Here's how the part is built. I have some questions about the finished solid (model axes, mm). A direction names the side the tool comes from. Coordinates: 2 decimals unless noted, no trailing zeros. Order: outer loops, then holes, each group sorted by start corner. A loop starts at its lowest first (then second) coordinate and runs counter-clockwise, first axis right, second up. Notation, with made-up numbers: (48.25, 58.25) - (77.25, 58.25) arc R20 cw to (77.25, 90.25) - close; hole circle Ø11 at (8, 27). An arc over 180 degrees is marked (long way). Answer as CSV lines item,"result". Start each with the question number.
Q1. I need wall thicknesses on line 1 (X direction, y = 17, z = -9.5); line 2 (X direction, y = 15.3, z = 0); line 3 (Z direction, x = 0, y = 15.3). Which ranges of each line are inside material? Lowest first, please.
Q2. Suppose I cut it at A-A (z = 0). Please give me the cut outline in (x, y), then the cut area to 3 significant figures.
Q3. Thinking about a two-plate mould opening in Z: for faces 1 (the face through (11, 18, 0)), 2 (the face through (14, 19, 0)), 3 (the face through (-2.44, 14.84, 0.54)), which applies, released by +Z, released by -Z, zero draft, split by the parting line, or undercut?
Q4. Suppose I cut it at C-C (x = 0). Please give me the cut outline in (y, z), then the cut area to 3 significant figures.
Q5. Suppose I cut it at D-D (y = 22.25). Please give me the cut outline in (x, z).
Q6. For pin 1 Ø6 at (x, z) = (0, 0) entering from +Y; pin 2 Ø4 at (x, z) = (1.5, -13.5) entering from +Y, each with a flat end and sliding along its axis, tell me the tip position at first contact or that it passes through.
Q7. For faces 4 (the face through (21.697, 25.494, 0.561)), 5 (the face through (-18, 21, 0)), which set-ups out of +Z, -Z, +X, -X, +Y, -Y let a thin tool reach every point of the face, with its end or its side?
Q8. Suppose I cut it at B-B (y = 8.5). Please give me the cut outline in (x, z), then the cut area to 3 significant figures.
from build123d import *

# Parameters (mm, degrees)
REVOLVE1_ANGLE            = 180
F_5_0MM_DOWEL_HOLE1_D     = 5
F_5_0MM_DOWEL_HOLE1_DEPTH = 6
F_5_0MM_DOWEL_HOLE1_TIP   = 1.502151548


with BuildPart() as part:
    # Sketch1 → Revolve1 (revolve, symmetric)
    with BuildSketch(Plane.XY) as revolve1_sk:
        Polygon((-25.5, 12.5), (25.5, 12.5), (25.5, 25.5), (18, 25.5), (18, 19), (11, 19), (11, 17.5), (-11, 17.5), (-11, 19), (-18, 19), (-18, 25.5), (-25.5, 25.5), align=None)
    revolve(axis=Axis((0, 0, 0), (1, 0, 0)), revolution_arc=REVOLVE1_ANGLE / 2)
    revolve(revolve1_sk.sketch, axis=Axis((0, 0, 0), (-1, 0, 0)), revolution_arc=REVOLVE1_ANGLE / 2)

    # Ø5.0mm Dowel Hole1
    with Locations(Plane.ZX.offset(17.5)):
        with Locations((0, 0)):
            Hole(F_5_0MM_DOWEL_HOLE1_D / 2, depth=F_5_0MM_DOWEL_HOLE1_DEPTH)
            with Locations((0, 0, -(F_5_0MM_DOWEL_HOLE1_DEPTH + F_5_0MM_DOWEL_HOLE1_TIP / 2))):  # 118° drill point
                Cone(0, F_5_0MM_DOWEL_HOLE1_D / 2, F_5_0MM_DOWEL_HOLE1_TIP, mode=Mode.SUBTRACT)


solid = part.part
Here are the results:
1,line 1,"x = -25.5 to -18, 18 to 25.5"
1,line 2,"x = -25.5 to -2.5, 2.5 to 25.5"
1,line 3,"z = -8.49 to -2.5, 2.5 to 8.49"
2,outline,"(-25.5, 12.5) - (-2.5, 12.5) - (-2.5, 17.5) - (-11, 17.5) - (-11, 19) - (-18, 19) - (-18, 25.5) - (-25.5, 25.5) - close; (2.5, 12.5) - (25.5, 12.5) - (25.5, 25.5) - (18, 25.5) - (18, 19) - (11, 19) - (11, 17.5) - (2.5, 17.5) - close"
2,area,"371 mm²"
3,face 1,"zero draft"
3,face 2,"split by the parting line"
3,face 3,"undercut"
4,outline,"(0, -17.5) arc R17.5 ccw to (17.32, -2.5) - (12.25, -2.5) arc R12.5 cw to (0, -12.5) - close; (0, 12.5) arc R12.5 cw to (12.25, 2.5) - (17.32, 2.5) arc R17.5 ccw to (0, 17.5) - close"
4,area,"210 mm²"
5,outline,"(-25.5, -12.46) - (-18, -12.46) - (-18, 12.46) - (-25.5, 12.46) - close; (18, -12.46) - (25.5, -12.46) - (25.5, 12.46) - (18, 12.46) - close"
6,pin 1,"stops at y = 17.5"
6,pin 2,"stops at y = 13.19"
7,face 4,"+X, -X, +Y"
7,face 5,"+Y"
8,outline,"(-25.5, -24.04) - (-18, -24.04) - (-18, -16.99) - (-11, -16.99) - (-11, -15.3) - (11, -15.3) - (11, -16.99) - (18, -16.99) - (18, -24.04) - (25.5, -24.04) - (25.5, -9.17) - (-25.5, -9.17) - close; (-25.5, 9.17) - (25.5, 9.17) - (25.5, 24.04) - (18, 24.04) - (18, 16.99) - (11, 16.99) - (11, 15.3) - (-11, 15.3) - (-11, 16.99) - (-18, 16.99) - (-18, 24.04) - (-25.5, 24.04) - close"
8,area,"935 mm²"
